Read the model definition and answer for the solid it produces. Units are mm, in the model's axes. Face numbers are marked on the shaded views. A direction names the side the tool comes from. Coordinates: 2 decimals unless noted, no trailing zeros. Write each loop counter-clockwise with the first axis right and the second up, starting at its lowest first coordinate (ties: lowest second). Pieces come first, ordered by that corner, then holes. Notation, with made-up numbers: (-29, 28.5) -> (-25, 28.5) arc R21 ccw to (-25, 59.5) -> close; hole circle Ø8 at (-31, 44). An arc over 180 degrees is marked (long way). Answer as a JSON object with one key per item and string values. Group by question number.
(1) Find section A-A (x = 16). Give the vertices of the cut face in (y, z).
(2) Flat-ended cylindrical pins translate along their axes: P1, Ø3, axis at x = 16.5, z = 25, coming from the +Y side; P2, Ø4.5, axis at x = 16, z = 9.34, coming from the -Y side; P3, Ø3, axis at y = 21, z = 20.5, coming from the +X side. Find the tip coordinate at first contact, or state that the pin passes through.
(3) Straight lines are drawn through the part: L1, parallel to X at y = 21, z = 10.75; L2, parallel to Z at x = 5, y = 3.75; L3, parallel to Y at x = 24, z = 18.5. For each, find the intervals that lie inside material, in ascending order.
(4) Find section B-B (x = 26.5). Give the vertices of the cut face in (y, z), then the cut area to 3 significant figures.
(5) Which of the six approach directions +Z, -Z, +X, -X, +Y, -Y give full straight-line access (tool end or side, diameter ignored) to the marked faces 1 and 2?
(6) Find section C-C (x = 23). Give the vertices of the cut face in (y, z), then the cut area to 3 significant figures.
(7) For a pull along Z with two mould halves and no side action, classify the marked faces 3, 4 and 5 as +Z half, -Z half, draft (parallel to the pull), parting line (faces both ways), or undercut.
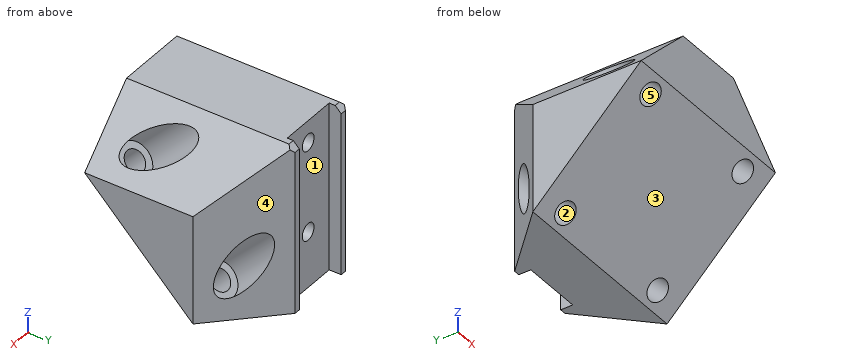
from build123d import *

# Parameters (mm, degrees)
SKETCH1_W           = 28
SKETCH1_H           = 28
BOSS_EXTRUDE1_DEPTH = 32
CHAMFER1_SIZE       = 18
SKETCH2_R           = 1.4
CUT_EXTRUDE1_DEPTH  = 5.5
CHAMFER2_SIZE       = 1
SKETCH3_R           = 1.8
CUT_EXTRUDE2_DEPTH  = 42.785164832
SKETCH4_R           = 3
CUT_EXTRUDE3_DEPTH  = 22
CHAMFER3_SIZE       = 10
SKETCH5_W           = 10
SKETCH5_H           = 28
CUT_EXTRUDE4_DEPTH  = 2


with BuildPart() as part:
    # Sketch1 → Boss-Extrude1 (new body)
    with BuildSketch(Plane(origin=(0, 0, 0), x_dir=(0, 0, -1), z_dir=(1, 0, 0))):
        with Locations((-14, 14)):
            Rectangle(SKETCH1_W, SKETCH1_H)
    extrude(amount=BOSS_EXTRUDE1_DEPTH)

    # Chamfer1
    chamfer1_edges = [part.edges().sort_by_distance(p)[0] for p in [
        (16, 0, 0),
    ]]
    chamfer(chamfer1_edges, length=CHAMFER1_SIZE)

    # Sketch2 → Cut-Extrude1 (cut)
    with BuildSketch(Plane(origin=(0, 28, 0), x_dir=(1, 0, 0), z_dir=(0, 1, 0))):
        with Locations(Location((16, -9.337953515, 0), (0, 0, 270))):
            Circle(SKETCH2_R)
        with Locations(Location((16, -24.337953515, 0), (0, 0, 270))):
            Circle(SKETCH2_R)
    extrude(amount=-CUT_EXTRUDE1_DEPTH, mode=Mode.SUBTRACT)

    # Chamfer2
    chamfer2_edges = [part.edges().sort_by_distance(p)[0] for p in [
        (16, 28, 28),
    ]]
    chamfer(chamfer2_edges, length=CHAMFER2_SIZE)

    # Sketch3 → Cut-Extrude2 (cut, through all)
    with BuildSketch(Plane(origin=(0, 9, 9), x_dir=(-1, 0, 0), z_dir=(0, -0.7071067811865487, -0.7071067811865465))):
        with Locations(Location((-5, -10, 0), (0, 0, 90))):
            Circle(SKETCH3_R)
        with Locations(Location((-27, -10, 0), (0, 0, 90))):
            Circle(SKETCH3_R)
        with Locations(Location((-27, 10, 0), (0, 0, 90))):
            Circle(SKETCH3_R)
        with Locations(Location((-5, 10, 0), (0, 0, 90))):
            Circle(SKETCH3_R)
    extrude(amount=-CUT_EXTRUDE2_DEPTH, mode=Mode.SUBTRACT)

    # Sketch4 → Cut-Extrude3 (cut)
    with BuildSketch(Plane(origin=(0, 27.5, 27.5), x_dir=(1, 0, 0), z_dir=(0, 0.7071067811865477, 0.7071067811865475))):
        with Locations(Location((5, 10, 0), (0, 0, 270))):
            Circle(SKETCH4_R)
        with Locations(Location((27, 10, 0), (0, 0, 270))):
            Circle(SKETCH4_R)
        with Locations(Location((27, -10, 0), (0, 0, 270))):
            Circle(SKETCH4_R)
        with Locations(Location((5, -10, 0), (0, 0, 270))):
            Circle(SKETCH4_R)
    extrude(amount=-CUT_EXTRUDE3_DEPTH, mode=Mode.SUBTRACT)

    # Chamfer3
    # the kernel refuses this chamfer: 10 mm, written as the material it takes off along each edge
    with BuildSketch(Plane(origin=(0, 28, 52.71682988), x_dir=(-0.027495876610586372, -0.9996219169112968, 0), z_dir=(0, 0, -1)), Plane(origin=(0, -25.71682988, 28), x_dir=(-0.027495876610586372, 0, -0.9996219169112968), z_dir=(0, 1, 0)), Plane(origin=(32, -25.71682988, 28), x_dir=(-0.9996219169112968, 0, 0.027495876610586317), z_dir=(0, 1, 0)), Plane(origin=(32, 28, 52.71682988), x_dir=(-0.9996219169112968, 0.027495876610586317, 0), z_dir=(0, 0, -1))) as chamfer3_piece_1:
        Polygon((CHAMFER3_SIZE * 0.999621916911, -CHAMFER3_SIZE * 0.0274958766106), (-CHAMFER3_SIZE * 0.0274958766106, -CHAMFER3_SIZE * 0.999621916911), (0, 0), align=None)
    extrude(amount=78.433659759, mode=Mode.SUBTRACT)

    # Sketch5 → Cut-Extrude4 (cut)
    with BuildSketch(Plane(origin=(0, 28, 0), x_dir=(1, 0, 0), z_dir=(0, 1, 0))):
        with Locations((15.986268974, -14)):
            Rectangle(SKETCH5_W, SKETCH5_H)
    extrude(amount=-CUT_EXTRUDE4_DEPTH, mode=Mode.SUBTRACT)


solid = part.part
Results below:
{
 "1": {"outline": "(0, 18) -> (18, 0) -> (26, 0) -> (26, 7.94) -> (22.5, 7.94) -> (22.5, 10.74) -> (26, 10.74) -> (26, 22.94) -> (22.5, 22.94) -> (22.5, 25.74) -> (26, 25.74) -> (26, 28) -> (0, 28) -> close"},
 "2": {"P1": "stops at y = 26", "P2": "stops at y = 6.41", "P3": "stops at x = 30.28"},
 "3": {"L1": "x = 3 to 3.81, 6.19 to 25.81, 28.19 to 29", "L2": "z = 14.25 to 15.35, 22.13 to 23", "L3": "y = 0 to 26"},
 "4": {"outline": "(0, 18) -> (0.71, 17.29) -> (3.65, 20.24) -> (2.78, 21.11) -> (5.17, 23.5) -> (0, 23.5) -> close; (3.15, 14.85) -> (14.85, 3.15) -> (17.79, 6.1) -> (16.92, 6.96) -> (23.5, 13.54) -> (23.5, 23.5) -> (13.54, 23.5) -> (6.96, 16.92) -> (6.1, 17.79) -> close; (17.29, 0.71) -> (18, 0) -> (23.5, 0) -> (23.5, 5.17) -> (21.11, 2.78) -> (20.24, 3.65) -> close", "area": "286 mm2"},
 "5": {"face 1": "+Z, -Z, +Y", "face 2": "none"},
 "6": {"outline": "(0, 18) -> (18, 0) -> (27, 0) -> (27, 27) -> (0, 27) -> close", "area": "567 mm2"},
 "7": {"face 3": "-Z half", "face 4": "draft", "face 5": "undercut"}
}
